Study the drawing (mm; zero at the part's minimum x, y, z) and answer. A direction names the side the tool comes from. Give positions to 0.01 mm unless a question says otherwise; leave off trailing zeros. Write each loop counter-clockwise with the first axis right and the second up, starting at its lowest first coordinate (ties: lowest second). Pieces come first, ordered by that corner, then holes. Notation, with made-up numbers: (-3, 1) -> (7, 1) arc R13 ccw to (7, 17) -> close; hole circle Ø9 at (15, -9.5). An arc over 180 degrees is marked (long way). One line per question, with ' | ' between items.
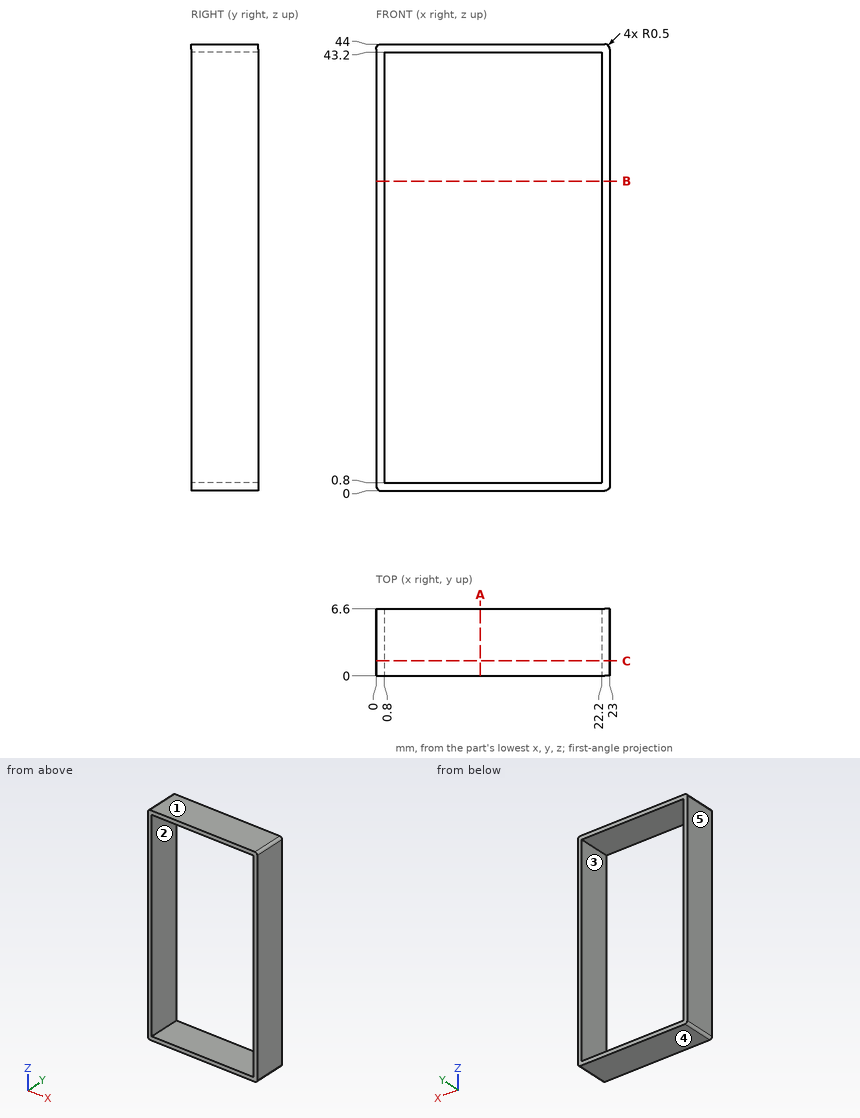
Item 1: A tool of negligible diameter and unlimited length cuts with its end or side. For the marked faces 1 and 2, from which of +Z, -Z, +X, -X, +Y, -Y can it reach the whole face along a straight path? Write none if from no direction.
Answers below:
face 1: +Z, +X, -X, +Y, -Y | face 2: +Y, -Y
Item 2: Find section A-A (x = 10.25). Write down the section's boundary in (y, z).
Answers below:
outline: (0, 0) -> (6.6, 0) -> (6.6, 0.8) -> (0, 0.8) -> close; (0, 43.2) -> (6.6, 43.2) -> (6.6, 44) -> (0, 44) -> close
Item 3: Determine the mould class of the marked faces 3, 4 and 5 for opening direction X: pulls with the +X half, pulls with the -X half, needs draft (parallel to the pull), parting line crosses it, or undercut.
Answers below:
face 3: undercut | face 4: needs draft | face 5: pulls with the -X half
Item 4: Find section B-B (z = 30.5). Write down the section's boundary in (x, y), then the cut area to 3 significant figures.
Answers below:
outline: (0, 0) -> (0.8, 0) -> (0.8, 6.6) -> (0, 6.6) -> close; (22.2, 0) -> (23, 0) -> (23, 6.6) -> (22.2, 6.6) -> close | area: 10.6 mm²
Item 5: Consider line 1 (X direction, y = 0.5, z = 36); line 2 (Z direction, x = 16.5, y = 3.25). Determine where each line is inside the solid, lowest interval first. Write a range as [from, to].
Answers below:
line 1: [0, 0.8], [22.2, 23] | line 2: [0, 0.8], [43.2, 44]
Item 6: Find section C-C (y = 1.5). Write down the section's boundary in (x, z), then the cut area to 3 significant figures.
Answers below:
outline: (0, 0.5) arc R0.5 ccw to (0.5, 0) -> (22.5, 0) arc R0.5 ccw to (23, 0.5) -> (23, 43.5) arc R0.5 ccw to (22.5, 44) -> (0.5, 44) arc R0.5 ccw to (0, 43.5) -> close; hole (0.8, 0.8) -> (22.2, 0.8) -> (22.2, 43.2) -> (0.8, 43.2) -> close | area: 104 mm²
